```python
from build123d import *

# Parameters (mm, degrees)
SKETCH1_R           = 2.999997759
SKETCH1_R_2         = 1.35
BOSS_EXTRUDE1_DEPTH = 2.54
SKETCH2_W           = 34.5908584
SKETCH2_H           = 10.2596717
BOSS_EXTRUDE2_DEPTH = 7.62
SKETCH3_W           = 5.570985132
SKETCH3_H           = 23.769243549
BOSS_EXTRUDE3_DEPTH = 7.62
SKETCH4_W           = 14.639482868
SKETCH4_H           = 13.879415804
BOSS_EXTRUDE4_DEPTH = 1.27
SKETCH5_R           = 1.180885515
BOSS_EXTRUDE5_DEPTH = 7.62
SKETCH6_R           = 2.837726638
SKETCH6_R_2         = 3.093496415
SKETCH6_R_3         = 2.974585048
BOSS_EXTRUDE6_DEPTH = 12.7


with BuildPart() as part:
    # Sketch1 → Boss-Extrude1 (new body)
    # profile 1 of 5: a face of its own
    with BuildSketch(Plane(origin=(0, 0, 0), x_dir=(1, 0, 0), z_dir=(0, 1, 0))):
        with BuildLine():
            Line((-39.500002241, -28), (39.500002241, -28))
            ThreePointArc((39.500002241, -28), (41.621321, -27.121321), (42.5, -25.000002241))
            Line((42.5, -25.000002241), (42.5, 25.000002241))
            ThreePointArc((42.5, 25.000002241), (41.621321, 27.121321), (39.500002241, 28))
            Line((39.500002241, 28), (-39.500002241, 28))
            ThreePointArc((-39.500002241, 28), (-41.621321, 27.121321), (-42.5, 25.000002241))
            Line((-42.5, 25.000002241), (-42.5, -25.000002241))
            ThreePointArc((-42.5, -25.000002241), (-41.621321, -27.121321), (-39.500002241, -28))
        make_face()
        with Locations((39, 24.5)):
            Circle(SKETCH1_R, mode=Mode.SUBTRACT)
        with Locations((-19, -24.5)):
            Circle(SKETCH1_R, mode=Mode.SUBTRACT)
        with Locations((-19, 24.5)):
            Circle(SKETCH1_R, mode=Mode.SUBTRACT)
        with Locations((39, -24.5)):
            Circle(SKETCH1_R, mode=Mode.SUBTRACT)
    # profile 2 of 5: a face of its own
    with BuildSketch(Plane(origin=(0, 0, 0), x_dir=(1, 0, 0), z_dir=(0, 1, 0))):
        with Locations((-19, 24.5)):
            Circle(SKETCH1_R)
        with Locations(Location((-19, 24.5, 0), (0, 0, 270))):
            Circle(SKETCH1_R_2, mode=Mode.SUBTRACT)
    # profile 3 of 5: a face of its own
    with BuildSketch(Plane(origin=(0, 0, 0), x_dir=(1, 0, 0), z_dir=(0, 1, 0))):
        with Locations((-19, -24.5)):
            Circle(SKETCH1_R)
        with Locations(Location((-19, -24.5, 0), (0, 0, 270))):
            Circle(SKETCH1_R_2, mode=Mode.SUBTRACT)
    # profile 4 of 5: a face of its own
    with BuildSketch(Plane(origin=(0, 0, 0), x_dir=(1, 0, 0), z_dir=(0, 1, 0))):
        with Locations((39, 24.5)):
            Circle(SKETCH1_R)
        with Locations(Location((39, 24.5, 0), (0, 0, 270))):
            Circle(SKETCH1_R_2, mode=Mode.SUBTRACT)
    # profile 5 of 5: a face of its own
    with BuildSketch(Plane(origin=(0, 0, 0), x_dir=(1, 0, 0), z_dir=(0, 1, 0))):
        with Locations((39, -24.5)):
            Circle(SKETCH1_R)
        with Locations(Location((39, -24.5, 0), (0, 0, 270))):
            Circle(SKETCH1_R_2, mode=Mode.SUBTRACT)
    extrude(amount=BOSS_EXTRUDE1_DEPTH)

    # Sketch2 → Boss-Extrude2 (add)
    with BuildSketch(Plane(origin=(0, 2.54, 0), x_dir=(1, 0, 0), z_dir=(0, 1, 0))):
        with Locations((6.499175034, -22.87016415)):
            Rectangle(SKETCH2_W, SKETCH2_H)
    extrude(amount=BOSS_EXTRUDE2_DEPTH)

    # Sketch3 → Boss-Extrude3 (add)
    with BuildSketch(Plane(origin=(0, 2.54, 0), x_dir=(1, 0, 0), z_dir=(0, 1, 0))):
        with Locations((-27.506444174, 3.193413678)):
            Rectangle(SKETCH3_W, SKETCH3_H)
    extrude(amount=BOSS_EXTRUDE3_DEPTH)

    # Sketch4 → Boss-Extrude4 (add)
    with BuildSketch(Plane(origin=(0, 2.54, 0), x_dir=(1, 0, 0), z_dir=(0, 1, 0))):
        with Locations((10.616389604, 7.997233107)):
            Rectangle(SKETCH4_W, SKETCH4_H)
    extrude(amount=BOSS_EXTRUDE4_DEPTH)

    # Sketch5 → Boss-Extrude5 (add)
    with BuildSketch(Plane(origin=(0, 2.54, 0), x_dir=(1, 0, 0), z_dir=(0, 1, 0))):
        with Locations(Location((-13.019538676, 24.586601174, 0), (0, 0, 270))):
            Circle(SKETCH5_R)
        with Locations(Location((-10.479538676, 24.586601174, 0), (0, 0, 270))):
            Circle(SKETCH5_R)
        with Locations(Location((-7.939538676, 24.586601174, 0), (0, 0, 270))):
            Circle(SKETCH5_R)
        with Locations(Location((-5.399538676, 24.586601174, 0), (0, 0, 270))):
            Circle(SKETCH5_R)
        with Locations(Location((-2.859538676, 24.586601174, 0), (0, 0, 270))):
            Circle(SKETCH5_R)
        with Locations(Location((-0.319538676, 24.586601174, 0), (0, 0, 270))):
            Circle(SKETCH5_R)
        with Locations(Location((2.220461324, 24.586601174, 0), (0, 0, 270))):
            Circle(SKETCH5_R)
        with Locations(Location((4.760461324, 24.586601174, 0), (0, 0, 270))):
            Circle(SKETCH5_R)
        with Locations(Location((7.300461324, 24.586601174, 0), (0, 0, 270))):
            Circle(SKETCH5_R)
    extrude(amount=BOSS_EXTRUDE5_DEPTH)

    # Sketch6 → Boss-Extrude6 (add)
    with BuildSketch(Plane(origin=(0, 2.54, 0), x_dir=(1, 0, 0), z_dir=(0, 1, 0))):
        with Locations(Location((-14.489308001, 14.172406875, 0), (0, 0, 90))):
            Circle(SKETCH6_R)
        with Locations(Location((-14.489308001, -0.87870872, 0), (0, 0, 90))):
            Circle(SKETCH6_R_2)
        with Locations(Location((27.833366931, 7.537539442, 0), (0, 0, 90))):
            Circle(SKETCH6_R_3)
    extrude(amount=BOSS_EXTRUDE6_DEPTH)


solid = part.part
```
The listing builds one solid part. Answer for the finished solid, in the listing's coordinates (mm). A direction names the side the tool comes from. Round coordinates to 2 decimals unless told otherwise and drop trailing zeros. Write each loop counter-clockwise with the first axis right and the second up, starting at its lowest first coordinate (ties: lowest second). Pieces come first, ordered by that corner, then holes. Notation, with made-up numbers: (9, 67) -> (33, 67) arc R14 cw to (33, 74) -> close; hole circle Ø11 at (-25, 40.5). An arc over 180 degrees is marked (long way). Use CSV: the item, a comma, the result in double quotes. Start each with the question number.
(1) Each of these flat-tipped pins is pushed along its axis until it touches: pin 1 (1.5 mm diameter, centred on y = 9, z = -10.5, fed in from -X); pin 2 (8.5 mm diameter, centred on y = 7.5, z = -8.5, fed in from +X); pin 3 (2.5 mm diameter, centred on x = -0.5, z = -24.5, fed in from +Y). Where does it stop, or does it pass through?
(2) Section C-C on y = 7.5 is taken. Count the separate pieces of the cut face and the enclosed holes in it, then the cut area to 3 significant figures.
(3) Section D-D on x = -28 is taken. Give the vertices of the cut face in (y, z), then the cut area to 3 significant figures.
(4) Section B-B on x = 10.5 is taken. Give the vertices of the cut face in (y, z).
(5) The mould has two halves that part along X. Classify faces 4 (the face through (42.5, 1, 0)), 5 (the face through (24.884, 8.801, -7.15)), 6 (the face through (6, 10.16, 23)): released by +X, released by -X, zero draft, split by the parting line, or undercut.
(6) Which of the six approach directions +Z, -Z, +X, -X, +Y, -Y give full straight-line access (tool end or side, diameter ignored) to faces 1 (the face through (23.795, 6, 23)), 2 (the face through (-12.968, 6.297, -25.766)), 3 (the face through (-30.292, 6, -3))?
(7) Consider L1, parallel to X at y = 0.55, z = -24.5; L2, parallel to Y at x = -22.5, z = 8; L3, parallel to X at y = 8, z = 21.5. Determine where each line is inside the solid, lowest interval first. Write a range as from..to.
(8) Section A-A on z = 5 is taken. Give the vertices of the cut face in (x, y).
A:
1,pin 1,"stops at x = -30.29"
1,pin 2,"stops at x = 30.81"
1,pin 3,"stops at y = 10.16"
2,separate pieces,"14"
2,enclosed holes,"0"
2,area,"610 mm²"
3,outline,"(0, -28) -> (2.54, -28) -> (2.54, -15.08) -> (10.16, -15.08) -> (10.16, 8.69) -> (2.54, 8.69) -> (2.54, 28) -> (0, 28) -> close"
3,area,"323 mm²"
4,outline,"(0, -28) -> (2.54, -28) -> (2.54, -14.94) -> (3.81, -14.94) -> (3.81, -1.06) -> (2.54, -1.06) -> (2.54, 17.74) -> (10.16, 17.74) -> (10.16, 28) -> (0, 28) -> close"
5,face 4,"released by +X"
5,face 5,"undercut"
5,face 6,"zero draft"
6,face 1,"+Z, -Z, +X, +Y"
6,face 2,"+Y"
6,face 3,"+Z, -Z, -X, +Y"
7,L1,"x = -42.5..-20.35, -17.65..37.65, 40.35..42.5"
7,L2,"y = 0..2.54"
7,L3,"x = -10.8..23.79"
8,outline,"(-42.5, 0) -> (42.5, 0) -> (42.5, 2.54) -> (-24.72, 2.54) -> (-24.72, 10.16) -> (-30.29, 10.16) -> (-30.29, 2.54) -> (-42.5, 2.54) -> close"
